from build123d import *

# Parameters (mm, degrees)
BOSS_EXTRU_1_DEPTH      = 27
ESQUISSE5_R             = 1.3
ENL_V_MAT_EXTRU_1_DEPTH = 18
ESQUISSE6_R             = 2.9
ENL_V_MAT_EXTRU_2_DEPTH = 3


with BuildPart() as part:
    # Esquisse1 → Boss.-Extru.1 (new body)
    with BuildSketch(Plane.XY):
        with BuildLine():
            Line((-12.560062385, 0), (-18.560062385, 0))
            Line((-18.560062385, 0), (-18.560062385, 18))
            Line((-18.560062385, 18), (18.560062385, 18))
            Line((18.560062385, 18), (18.560062385, 0))
            Line((18.560062385, 0), (12.560062385, 0))
            ThreePointArc((12.560062385, 0), (0, 12.560062385), (-12.560062385, 0))
        make_face()
    extrude(amount=BOSS_EXTRU_1_DEPTH)

    # Esquisse5 → Enlèv. mat.-Extru.1 (cut)
    with BuildSketch(Plane(origin=(0, 18, 0), x_dir=(1, 0, 0), z_dir=(0, 1, 0))):
        with Locations((15.560062385, -3)):
            Circle(ESQUISSE5_R)
        with Locations((15.560062385, -24)):
            Circle(ESQUISSE5_R)
        with Locations((-15.560062385, -3)):
            Circle(ESQUISSE5_R)
        with Locations((-15.560062385, -24)):
            Circle(ESQUISSE5_R)
    extrude(amount=-ENL_V_MAT_EXTRU_1_DEPTH, mode=Mode.SUBTRACT)

    # Esquisse6 → Enlèv. mat.-Extru.2 (cut)
    with BuildSketch(Plane(origin=(0, 18, 0), x_dir=(1, 0, 0), z_dir=(0, 1, 0))):
        with Locations((15.560062385, -3)):
            Circle(ESQUISSE6_R)
        with Locations((15.560062385, -24)):
            Circle(ESQUISSE6_R)
        with Locations((-15.560062385, -3)):
            Circle(ESQUISSE6_R)
        with Locations((-15.560062385, -24)):
            Circle(ESQUISSE6_R)
    extrude(amount=-ENL_V_MAT_EXTRU_2_DEPTH, mode=Mode.SUBTRACT)


solid = part.part
Work out the finished part from the listing and answer in its coordinate system (mm). A direction names the side the tool comes from. Coordinates: 2 decimals unless noted, no trailing zeros. Write each loop counter-clockwise with the first axis right and the second up, starting at its lowest first coordinate (ties: lowest second). Pieces come first, ordered by that corner, then holes.
1. For faces 4 (the cylindrical face through (-16.86, 7.6, 2.94)), 5 (the cylindrical face through (-17.861, 16.521, 25.765)), determine the directions among +Z, -Z, +X, -X, +Y, -Y from which every point of the face is accessible in a straight line to the end or side of a thin tool.
Results list:
face 4: +Y, -Y
face 5: +Y
2. Consider line 1 along Z through (x, y) = (15.5, 3.75); line 2 along X through (y, z) = (8.25, 24); line 3 along Z through (x, y) = (15, 17). Determine where each line is inside the solid, lowest interval first.
Results list:
line 1: z = 0 to 1.7, 4.3 to 22.7, 25.3 to 27
line 2: x = -18.56 to -16.86, -14.26 to -9.47, 9.47 to 14.26, 16.86 to 18.56
line 3: z = 0 to 0.15, 5.85 to 21.15, 26.85 to 27
3. The part is cut by section D-D, the plane y = 3.5. Write down the section's boundary in (x, z), and give its area (3 significant figures).
Results list:
outline: (-18.56, 0) - (-12.06, 0) - (-12.06, 27) - (-18.56, 27) - close; (12.06, 0) - (18.56, 0) - (18.56, 27) - (12.06, 27) - close; hole circle Ø2.6 at (-15.56, 3); hole circle Ø2.6 at (-15.56, 24); hole circle Ø2.6 at (15.56, 3); hole circle Ø2.6 at (15.56, 24)
area: 330 mm2
4. The part is cut by section A-A, the plane y = 14.5. Write down the section's boundary in (x, z).
Results list:
outline: (-18.56, 0) - (18.56, 0) - (18.56, 27) - (-18.56, 27) - close; hole circle Ø2.6 at (-15.56, 3); hole circle Ø2.6 at (-15.56, 24); hole circle Ø2.6 at (15.56, 3); hole circle Ø2.6 at (15.56, 24)
5. The part is cut by section B-B, the plane z = 24. Write down the section's boundary in (x, y), and give its area (3 significant figures).
Results list:
outline: (-18.56, 0) - (-16.86, 0) - (-16.86, 15) - (-18.46, 15) - (-18.46, 18) - (-18.56, 18) - close; (-14.26, 0) - (-12.56, 0) arc R12.56 cw to (12.56, 0) - (14.26, 0) - (14.26, 15) - (12.66, 15) - (12.66, 18) - (-12.66, 18) - (-12.66, 15) - (-14.26, 15) - close; (16.86, 0) - (18.56, 0) - (18.56, 18) - (18.46, 18) - (18.46, 15) - (16.86, 15) - close
area: 308 mm2
6. A flat-ended cylindrical pin translates along its axis: pin 1 (3.5 mm diameter, centred on x = -15.56, z = 3, fed in from +Y). Find the tip coordinate at first contact, or state that the pin passes through.
Results list:
pin 1: stops at y = 15
7. The part is cut by section C-C, the plane x = -15. Write down the section's boundary in (y, z).
Results list:
outline: (0, 0) - (18, 0) - (18, 0.15) - (15, 0.15) - (15, 1.83) - (0, 1.83) - close; (0, 4.17) - (15, 4.17) - (15, 5.85) - (18, 5.85) - (18, 21.15) - (15, 21.15) - (15, 22.83) - (0, 22.83) - close; (0, 25.17) - (15, 25.17) - (15, 26.85) - (18, 26.85) - (18, 27) - (0, 27) - close
8. For a pull along X with two mould halves and no side action, classify faces 1 (the flat face through (0, 13, 0)), 2 (the cylindrical face through (-17.7, 16.52, 1.04)), 3 (the flat face through (18.56, 9, 13)) as +X half, -X half, draft (parallel to the pull), parting line (faces both ways), or undercut.
Results list:
face 1: draft
face 2: undercut
face 3: +X half
